from build123d import *

# Parameters (mm, degrees)
F0_W     = 774.7
F0_H     = 76.2
F1_DEPTH = 5.9944
F2_R     = 6.35
F3_DEPTH = 11.9888
F4_R     = 6.35
F5_DEPTH = 11.9888
F6_W     = 596.9
F6_H     = 76.2
F7_DEPTH = 11.9888


with BuildPart() as f1:
    # F0 (on Top) → F1 (new body, symmetric)
    with BuildSketch(Plane.XY):
        Rectangle(F0_W, F0_H)
    extrude(amount=F1_DEPTH, both=True)

    # F2 (on face) → F3 (cut, through all)
    with BuildSketch(Plane(origin=(0, 0, -5.9944), x_dir=(1, 0, 0), z_dir=(0, 0, -1))):
        with Locations((-316.70625, 0)):
            Circle(F2_R)
        with Locations((323.85, 0)):
            Circle(F2_R)
    extrude(amount=-F3_DEPTH, mode=Mode.SUBTRACT)

    # F4 (on face) → F5 (cut, through all)
    with BuildSketch(Plane.XY.offset(5.9944)):
        with Locations((-349.25, 0)):
            Circle(F4_R)
        with Locations((-234.95, 0)):
            Circle(F4_R)
    extrude(amount=-F5_DEPTH, mode=Mode.SUBTRACT)

    # F6 (on face) → F7 (cut, through all)
    with BuildSketch(Plane.XY.offset(5.9944)):
        with Locations((88.9, 0)):
            Rectangle(F6_W, F6_H)
    extrude(amount=-F7_DEPTH, mode=Mode.SUBTRACT)


solid = f1.part
The model under review builds one solid part; all positions refer to its coordinate system, in mm. Round coordinates to 2 decimals unless told otherwise and drop trailing zeros. Order: outer loops, then holes, each group sorted by start corner. A loop starts at its lowest first (then second) coordinate and runs counter-clockwise, first axis right, second up. Notation, with made-up numbers: (54.5, -33.75) -> (82.5, -33.75) arc R31 ccw to (82.5, 3.25) -> close; hole circle Ø1 at (-27.75, 89.5). An arc over 180 degrees is marked (long way). Write item = value, one per line. Start each with the question number.
Item 1: Consider section B-B on z = 0.75. Write out the cut boundary in (x, y).
Item 2: For line 1 along Y through (x, z) = (-349.25, 3); line 2 along X through (y, z) = (3, 1); line 3 along Y through (x, z) = (-313.5, 3.5), list the stretches that pass through material, from the lowest coordinate up.
Item 3: Mouldability with a two-part tool opening along X and no side actions: class faces 1 (the face through (-355.594, 0.279, 0.084)), 2 (the face through (-300, 1, -5.994)), 3 (the face through (-387.35, -1, 0)) as released by +X, released by -X, zero draft, split by the parting line, or undercut.
Item 4: Consider section C-C on x = -234.95. Write out the cut boundary in (y, z).
Item 5: Consider section A-A on y = 0. Write out the cut boundary in (x, z), plus the area to 3 significant figures.
Item 6: Clearance check with a flat-ended pin moving along its axis: pin 1 Ø7.5 at (x, y) = (-234.95, 0) entering from +Z. State where the tip first meets the part, or that it passes through.
Item 7: Consider section D-D on x = -316. Write out the cut boundary in (y, z).
Conclusion:
q1.outline = (-387.35, -38.1) -> (-209.55, -38.1) -> (-209.55, 38.1) -> (-387.35, 38.1) -> close; hole circle Ø12.7 at (-349.25, 0); hole circle Ø12.7 at (-316.71, 0); hole circle Ø12.7 at (-234.95, 0)
q2.line_1 = -38.1 to -6.35, 6.35 to 38.1
q2.line_2 = -387.35 to -354.85, -343.65 to -322.3, -311.11 to -240.55, -229.35 to -209.55
q2.line_3 = -38.1 to -5.48, 5.48 to 38.1
q3.face_1 = undercut
q3.face_2 = zero draft
q3.face_3 = released by -X
q4.outline = (-38.1, -5.99) -> (-6.35, -5.99) -> (-6.35, 5.99) -> (-38.1, 5.99) -> close; (6.35, -5.99) -> (38.1, -5.99) -> (38.1, 5.99) -> (6.35, 5.99) -> close
q5.outline = (-387.35, -5.99) -> (-355.6, -5.99) -> (-355.6, 5.99) -> (-387.35, 5.99) -> close; (-342.9, -5.99) -> (-323.06, -5.99) -> (-323.06, 5.99) -> (-342.9, 5.99) -> close; (-310.36, -5.99) -> (-241.3, -5.99) -> (-241.3, 5.99) -> (-310.36, 5.99) -> close; (-228.6, -5.99) -> (-209.55, -5.99) -> (-209.55, 5.99) -> (-228.6, 5.99) -> close
q5.area = 1,670 mm2
q6.pin_1 = through
q7.outline = (-38.1, -5.99) -> (-6.31, -5.99) -> (-6.31, 5.99) -> (-38.1, 5.99) -> close; (6.31, -5.99) -> (38.1, -5.99) -> (38.1, 5.99) -> (6.31, 5.99) -> close
